```python
from build123d import *

# Parameters (mm, degrees)
SKETCH1_W           = 152.4
SKETCH1_H           = 50.8
BOSS_EXTRUDE1_DEPTH = 6.35
SKETCH2_R           = 20
CUT_EXTRUDE1_DEPTH  = 5.08
SKETCH3_R           = 15
CUT_EXTRUDE2_DEPTH  = 81.48233595
SKETCH5_R           = 2.15265
CUT_EXTRUDE4_DEPTH  = 25.4


with BuildPart() as part:
    # Sketch1 → Boss-Extrude1 (new body)
    with BuildSketch(Plane(origin=(0, 0, 0), x_dir=(1, 0, 0), z_dir=(0, 1, 0))):
        Rectangle(SKETCH1_W, SKETCH1_H)
    extrude(amount=-BOSS_EXTRUDE1_DEPTH)

    # Sketch2 → Cut-Extrude1 (cut)
    with BuildSketch(Plane(origin=(0, 0, 0), x_dir=(1, 0, 0), z_dir=(0, 1, 0))):
        with Locations(Location((0, 0, 0), (0, 0, 270))):
            Circle(SKETCH2_R)
    extrude(amount=-CUT_EXTRUDE1_DEPTH, mode=Mode.SUBTRACT)

    # Sketch3 → Cut-Extrude2 (cut, through all)
    with BuildSketch(Plane(origin=(0, -5.08, 0), x_dir=(1, 0, 0), z_dir=(0, 1, 0))):
        with Locations(Location((0, 0, 0), (0, 0, 270))):
            Circle(SKETCH3_R)
    extrude(amount=-CUT_EXTRUDE2_DEPTH, mode=Mode.SUBTRACT)

    # Sketch5 → Cut-Extrude4 (cut)
    with BuildSketch(Plane.ZY.offset(76.2)):
        with Locations((0, -3.175)):
            Circle(SKETCH5_R)
        with Locations((19.05, -3.175)):
            Circle(SKETCH5_R)
        with Locations(Location((-19.05, -3.175, 0), (0, 0, 180))):
            Circle(SKETCH5_R)
    cut_extrude4 = extrude(amount=-CUT_EXTRUDE4_DEPTH, mode=Mode.SUBTRACT)

    # Mirror1: Cut-Extrude4 across plane
    add(cut_extrude4.mirror(Plane(origin=(0, 0, 0), x_dir=(0, 0, 1), z_dir=(1, 0, 0))), mode=Mode.SUBTRACT)


solid = part.part
```
Here's how the part is built. I have some questions about the finished solid (model axes, mm). A direction names the side the tool comes from. Coordinates: 2 decimals unless noted, no trailing zeros. Order: outer loops, then holes, each group sorted by start corner. A loop starts at its lowest first (then second) coordinate and runs counter-clockwise, first axis right, second up.
1) We'd pull the mould along Y, two halves only. Please class faces 1 (the face through (-1, -3, -25.4)), 2 (the face through (50.8, -3, -19)), 3 (the face through (16, -6.35, 0)): +Y half, -Y half, draft (parallel to the pull), parting line (faces both ways), or undercut.
2) Imagine slicing it at C-C on x = -61.5. List the corners of the cut face in (y, z) for me (3 decimals).
3) Which directions (+Z, -Z, +X, -X, +Y, -Y) give clear straight access to the entire face, cutting with the end or side of a thin tool? Please do faces 4 (the face through (63.68, -1.04, -0.28)), 5 (the face through (-1, -3, 25.4)), 6 (the face through (-63.68, -2.35, -21.04)).
4) Imagine slicing it at A-A on z = 0. List the corners of the cut face in (x, y) for me.
5) Imagine slicing it at B-B on x = 0. List the corners of the cut face in (y, z) for me.
6) I need wall thicknesses on line 1 (X direction, y = -0.75, z = 0); line 2 (Z direction, x = -52.5, y = -3); line 3 (Z direction, x = -63.5, y = -1.75). Which ranges of each line are inside material? Lowest first, please.
7) Will these pins go through, and if not, where does the flat tip stop? pin 1 (12 mm diameter, centred on x = 1, z = -9.5, fed in from -Y); pin 2 (1.3 mm diameter, centred on y = -3, z = -0.5, fed in from +X); pin 3 (2 mm diameter, centred on y = -3.5, z = -0.5, fed in from -X).
Response values:
1. face 1: draft
1. face 2: undercut
1. face 3: -Y half
2. outline: (-6.35, -25.4) - (0, -25.4) - (0, 25.4) - (-6.35, 25.4) - close; hole circle Ø4.305 at (-3.175, -19.05); hole circle Ø4.305 at (-3.175, 0); hole circle Ø4.305 at (-3.175, 19.05)
3. face 4: +X
3. face 5: +Z, +X, -X, +Y, -Y
3. face 6: -X
4. outline: (-76.2, -6.35) - (-15, -6.35) - (-15, -5.08) - (-20, -5.08) - (-20, 0) - (-76.2, 0) - (-76.2, -1.02) - (-50.8, -1.02) - (-50.8, -5.33) - (-76.2, -5.33) - close; (15, -6.35) - (76.2, -6.35) - (76.2, -5.33) - (50.8, -5.33) - (50.8, -1.02) - (76.2, -1.02) - (76.2, 0) - (20, 0) - (20, -5.08) - (15, -5.08) - close
5. outline: (-6.35, -25.4) - (0, -25.4) - (0, -20) - (-5.08, -20) - (-5.08, -15) - (-6.35, -15) - close; (-6.35, 15) - (-5.08, 15) - (-5.08, 20) - (0, 20) - (0, 25.4) - (-6.35, 25.4) - close
6. line 1: x = -76.2 to -20, 20 to 76.2
6. line 2: z = -25.4 to -21.2, -16.9 to -2.15, 2.15 to 16.9, 21.2 to 25.4
6. line 3: z = -25.4 to -20.66, -17.44 to -1.61, 1.61 to 17.44, 20.66 to 25.4
7. pin 1: stops at y = -6.35
7. pin 2: stops at x = 50.8
7. pin 3: stops at x = -50.8
